```python
from build123d import *

# Parameters (mm, degrees)
BOSS_EXTRUDE1_DEPTH            = 25
CONVERT_SOLID1_START           = -1.51892
CONVERT_SOLID1_OUTLINE_W       = 184.752086141
CONVERT_SOLID1_OUTLINE_H       = 50
CONVERT_SOLID1_DEPTH           = 0.01892
EDGE_FLANGE1_STRIP_W           = 9.88568
EDGE_FLANGE1_STRIP_H           = 1.51892
EDGE_FLANGE1_STRIP_CUT_DEPTH   = 184.752086141
EDGE_FLANGE1_STRIP_2_W         = 9.88568
EDGE_FLANGE1_STRIP_2_H         = 1.51892
EDGE_FLANGE1_STRIP_CUT_2_DEPTH = 184.752086141
EDGE_FLANGE1_DEPTH             = 184.752086141
EDGE_FLANGE1_BEND_DEPTH        = 184.752086141
CUT_EXTRUDE2_DEPTH             = 197.424354221
CUT_EXTRUDE2_DEPTH_BACK        = 197.424354221
SKETCH13_R                     = 1.6


# Read off the part's stored shape, not the designer's step: Convert-Solid1
# Sheet-metal steps are written as plain solids
with BuildPart() as part:
    # Sketch2 → Boss-Extrude1 (new, symmetric)
    with BuildSketch(Plane.XY):
        Polygon((0, 0), (160, -92.37604307), (159.25, -93.675081176), (-0.75, -1.299038106), align=None)
    extrude(amount=BOSS_EXTRUDE1_DEPTH, both=True)

    # Convert-Solid1 outline → Convert-Solid1 (add)
    with BuildSketch(Plane(origin=(0, 0, 0), x_dir=(0.866025403784438, -0.500000000000001, 0), z_dir=(0.500000000000001, 0.866025403784438, 0)).offset(CONVERT_SOLID1_START)):
        with Locations((92.376043071, 0)):
            Rectangle(CONVERT_SOLID1_OUTLINE_W, CONVERT_SOLID1_OUTLINE_H)
    extrude(amount=CONVERT_SOLID1_DEPTH)

    # Edge-Flange1 strip (across the edge) → Edge-Flange1 strip cut (cut)
    with BuildSketch(Plane(origin=(160, -92.37604307, -25), x_dir=(0, 0, 1), z_dir=(-0.866025403784438, 0.5000000000000011, 0))):
        with Locations((-1.51892, -0.75946)):
            Rectangle(EDGE_FLANGE1_STRIP_W, EDGE_FLANGE1_STRIP_H)
    extrude(amount=EDGE_FLANGE1_STRIP_CUT_DEPTH, mode=Mode.SUBTRACT)

    # Edge-Flange1 strip 2 (across the edge) → Edge-Flange1 strip cut 2 (cut)
    with BuildSketch(Plane(origin=(0, 0, 25), x_dir=(0, 0, -1), z_dir=(0.866025403784438, -0.5000000000000011, 0))):
        with Locations((-1.51892, -0.75946)):
            Rectangle(EDGE_FLANGE1_STRIP_2_W, EDGE_FLANGE1_STRIP_2_H)
    extrude(amount=EDGE_FLANGE1_STRIP_CUT_2_DEPTH, mode=Mode.SUBTRACT)

    # Edge-Flange1 section (across the edge) → Edge-Flange1 (add)
    with BuildSketch(Plane(origin=(160, -92.37604307, -25), x_dir=(0, 0, 1), z_dir=(-0.866025403784438, 0.5000000000000011, 0))):
        with BuildLine():
            Line((0, 1.905), (0, 10.48108))
            Line((0, 10.48108), (1.51892, 10.48108))
            Line((1.51892, 10.48108), (1.51892, 1.905))
            ThreePointArc((1.51892, 1.905), (2.076881582, 0.557961582), (3.42392, 0))
            Line((3.42392, 0), (3.42392, -1.51892))
            ThreePointArc((3.42392, -1.51892), (1.00284295, -0.51607705), (0, 1.905))
        make_face()
    extrude(amount=EDGE_FLANGE1_DEPTH)

    # Edge-Flange1 section 2 (across the edge) → Edge-Flange1 bend (add)
    with BuildSketch(Plane(origin=(0, 0, 25), x_dir=(0, 0, -1), z_dir=(0.866025403784438, -0.5000000000000011, 0))):
        with BuildLine():
            Line((0, 1.905), (0, 10.48108))
            Line((0, 10.48108), (1.51892, 10.48108))
            Line((1.51892, 10.48108), (1.51892, 1.905))
            ThreePointArc((1.51892, 1.905), (2.076881582, 0.557961582), (3.42392, 0))
            Line((3.42392, 0), (3.42392, -1.51892))
            ThreePointArc((3.42392, -1.51892), (1.00284295, -0.51607705), (0, 1.905))
        make_face()
    extrude(amount=EDGE_FLANGE1_BEND_DEPTH)

    # Sketch13 → Cut-Extrude2 (cut, two sides: drawn at the far end of the back side and taken through both)
    with BuildSketch(Plane.XY.offset(25).offset(-CUT_EXTRUDE2_DEPTH_BACK)):
        with Locations(Location((9.743082385, 1.215259675, 0), (0, 0, 90))):
            Circle(SKETCH13_R)
    extrude(amount=CUT_EXTRUDE2_DEPTH + CUT_EXTRUDE2_DEPTH_BACK, mode=Mode.SUBTRACT)


solid = part.part
```
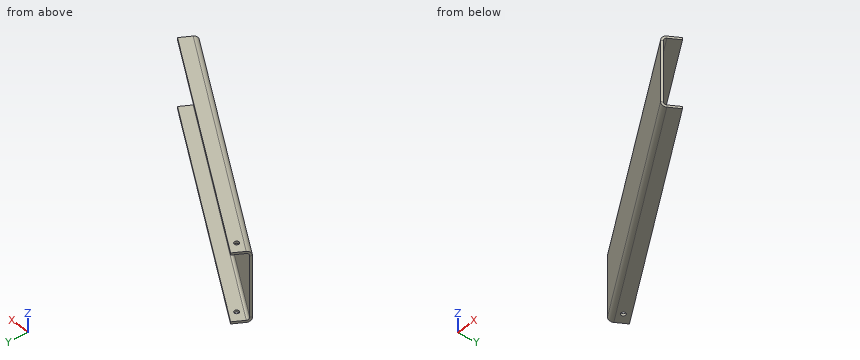
CAD build for the part. Positions are in the model's coordinates, mm. Give positions to 0.01 mm unless a question says otherwise; leave off trailing zeros. Loops run counter-clockwise (first coordinate to the right, second up) from the corner with the lowest first, then second, coordinate; pieces in that order, holes last. Notation, with made-up numbers: (18, 45.5) - (75, 45.5) arc R37 ccw to (75, 81.5) - close; hole circle Ø1 at (55, 56). An arc over 180 degrees is marked (long way). Put each result on its own line as item: value.
Q1. Flat gauge pins, fed straight in: pin 1 (1.5 mm diameter, centred on x = 146.5, z = 19, fed in from -Y); pin 2 (12 mm diameter, centred on y = -22.5, z = -16, fed in from -X); pin 3 (1.5 mm diameter, centred on x = 73, z = 4, fed in from -Y); pin 4 (4 mm diameter, centred on x = 9.74, y = 1.22, fed in from +Z). Where does each tip first touch, or does it go through?
Filled in:
pin 1: stops at y = -86.77
pin 2: stops at x = 25.54
pin 3: stops at y = -44.33
pin 4: stops at z = 25
Q2. Probe line 1 along X through (y, z) = (-86.5, -21); line 2 along Y through (x, z) = (38.5, -18); line 3 along X through (y, z) = (-83.5, -11). List the from-to ranges inside material, lowest first.
Filled in:
line 1: x = 146.78 to 149.82
line 2: y = -23.98 to -22.23
line 3: x = 141.59 to 144.63
Q3. Slice it at A-A (z = 0.5). Give the cut face in (x, y).
Filled in:
outline: (-0.76, -1.32) - (159.24, -93.69) - (160, -92.38) - (0, 0) - close
